Part model, mm, in its own coordinate system. A direction names the side the tool comes from. Round coordinates to 2 decimals unless told otherwise and drop trailing zeros. Loops run counter-clockwise (first coordinate to the right, second up) from the corner with the lowest first, then second, coordinate; pieces in that order, holes last.
(1) Cut at B-B on y = -24.25. List the corners of the cut face in (x, z).
(2) Mould opens along X. For faces 6 (the face through (-1.377, -16.901, 0.641)), 7 (the face through (-11, -18.5, 1)), 8 (the face through (-42.05, -4, -4)) say: +X half, -X half, draft (parallel to the pull), parting line (faces both ways), or undercut.
(3) Cut at D-D on x = -38. List the corners of the cut face in (y, z), then the cut area to 3 significant figures.
(4) Tool access for faces 1 (the face through (-33.938, -4, -4)), 2 (the face through (-40, -8.5, -4)), 3 (the face through (-49.732, -25, 1)), 4 (the face through (-43.48, -5.12, 6.23)), 5 (the face through (-31, -4, -9)): list every direction of +Z, -Z, +X, -X, +Y, -Y with a clear straight run to the whole face (end or side of a thin tool).
(5) Probe probe 1 along X at (y, z) = (-2.75, -7); probe 2 along X at (y, z) = (-3.5, 4); probe 3 along Z at (x, y) = (-55, -14). List the from-to ranges inside material, lowest first.
(6) Flat gauge pins, fed straight in: pin 1 (4 mm diameter, centred on x = -2, z = -6.5, fed in from -Y); pin 2 (1.5 mm diameter, centred on x = -37.5, z = 6, fed in from +Y); pin 3 (14 mm diameter, centred on x = -22, y = -20, fed in from -Z); pin 4 (2.5 mm diameter, centred on y = -4.5, z = -6.5, fed in from +X). Where does each tip first touch, or does it go through?
(7) Cut at A-A on z = -3.25. List the corners of the cut face in (x, y), then the cut area to 3 significant figures.
(8) Cut at C-C on z = 4.75. List the corners of the cut face in (x, y), then the cut area to 3 significant figures.
from build123d import *

# Parameters (mm, degrees)
EXTRUDE_1_DEPTH     = 1.3
SKETCH_2_R          = 6.1271e-05
SKETCH_2_R_2        = 1.854699803
CUT_EXTRUDE_1_DEPTH = 1.3
SKETCH_3_W          = 5
SKETCH_3_H          = 8.5
EXTRUDE_2_DEPTH     = 9
SKETCH_4_W          = 22.322793398
SKETCH_4_H          = 7.656611546
EXTRUDE_3_DEPTH     = 6
SKETCH_7_R          = 2.060894962
SKETCH_7_R_2        = 0.009430026
EXTRUDE_6_DEPTH     = 1.3
SKETCH_9_R          = 1.766576119
SKETCH_9_R_2        = 1.77
CUT_EXTRUDE_4_DEPTH = 13.5
SKETCH_11_R         = 2.5
EXTRUDE_7_DEPTH     = 10
SKETCH_5_R          = 3.177873229
EXTRUDE_4_DEPTH     = 10


with BuildPart() as part:
    # 草图1 → 凸台-拉伸1 (new body)
    with BuildSketch(Plane.XY):
        Polygon((-20.731582571, -20.531304637), (-20.731582571, -28.5), (-49.731582571, -28.5), (-49.731582571, -20.531304637), (-52.024986974, -18.5), (-67.347016347, -18.5), (-70.5, -15.347016347), (-70.5, 0), (0, 0), (0, -15.347016347), (-2.792647606, -18.5), (-18.700277933, -18.5), align=None)
    extrude(amount=EXTRUDE_1_DEPTH)

    # 草图2 → 切除-拉伸1 (cut)
    with BuildSketch(Plane(origin=(-0.901876225, 0, 0), x_dir=(-1, 0, 0), z_dir=(0, 0, -1))):
        with Locations((38.822404022, -18.263145779)):
            Circle(SKETCH_2_R)
        with Locations((24.094803283, -18.263145779)):
            Circle(SKETCH_2_R_2)
    extrude(amount=-CUT_EXTRUDE_1_DEPTH, mode=Mode.SUBTRACT)

    # 草图3 → 凸台-拉伸2 (add)
    with BuildSketch(Plane(origin=(0, 0, 0), x_dir=(-1, 0, 0), z_dir=(0, 0, -1))):
        with Locations((2.5, -4.25)):
            Rectangle(SKETCH_3_W, SKETCH_3_H)
        with Locations((31.437833881, -4.25)):
            Rectangle(SKETCH_3_W, SKETCH_3_H)
        with Locations((39.549598659, -4.25)):
            Rectangle(SKETCH_3_W, SKETCH_3_H)
        with Locations((67.475480729, -4.25)):
            Rectangle(SKETCH_3_W, SKETCH_3_H)
    extrude(amount=EXTRUDE_2_DEPTH)

    # 草图4 → 凸台-拉伸3 (add)
    with BuildSketch(Plane.XY.offset(1.3)):
        with Locations((-35.107201512, -24.671694227)):
            Rectangle(SKETCH_4_W, SKETCH_4_H)
    extrude(amount=EXTRUDE_3_DEPTH)

    # 草图7 → 凸台-拉伸6 (add)
    with BuildSketch(Plane(origin=(0, 0, 0), x_dir=(-1, 0, 0), z_dir=(0, 0, -1))):
        with Locations((24.996679508, -18.263145779)):
            Circle(SKETCH_7_R)
        with Locations((22.922712851, -19.688356139)):
            Circle(SKETCH_7_R_2)
    extrude(amount=-EXTRUDE_6_DEPTH)

    # 草图9 → 切除-拉伸4 (cut)
    with BuildSketch(Plane(origin=(0, 0, 0), x_dir=(-1, 0, 0), z_dir=(0, 0, -1))):
        with Locations((22.486064791, -16.932374865)):
            Circle(SKETCH_9_R)
        with Locations((47.612418274, -17.394192754)):
            Circle(SKETCH_9_R_2)
    extrude(amount=-CUT_EXTRUDE_4_DEPTH, mode=Mode.SUBTRACT)

    # 草图11 → 凸台-拉伸7 (add)
    with BuildSketch(Plane.XY.offset(1.3)):
        with Locations((-7.049667213, -4.299078236)):
            Circle(SKETCH_11_R)
        with Locations((-25.10539175, -4.501377507)):
            Circle(SKETCH_11_R)
        with Locations((-45.789989635, -4.160939668)):
            Circle(SKETCH_11_R)
        with Locations((-62.923589595, -4.217113271)):
            Circle(SKETCH_11_R)
    extrude(amount=EXTRUDE_7_DEPTH)

    # 草图5 → 凸台-拉伸4 (add)
    with BuildSketch(Plane.XY.offset(1.3)):
        with Locations((-60.836996038, -4.474043661)):
            Circle(SKETCH_5_R)
    extrude(amount=EXTRUDE_4_DEPTH)


solid = part.part
Final values:
1. outline: (-49.73, 0) - (-20.73, 0) - (-20.73, 1.3) - (-23.95, 1.3) - (-23.95, 7.3) - (-46.27, 7.3) - (-46.27, 1.3) - (-49.73, 1.3) - close
2. face 6: +X half
2. face 7: draft
2. face 8: undercut
3. outline: (-28.5, 0) - (-8.5, 0) - (-8.5, -9) - (0, -9) - (0, 1.3) - (-20.84, 1.3) - (-20.84, 7.3) - (-28.5, 7.3) - close
3. area: 159 mm2
4. face 1: -Z, +Y, -Y
4. face 2: -Z, +X, -X, -Y
4. face 3: +Z, -Z, -X, -Y
4. face 4: +Z
4. face 5: -Z, +X, -X, +Y, -Y
5. probe 1: x = -69.98 to -64.98, -42.05 to -37.05, -33.94 to -28.94, -5 to 0
5. probe 2: x = -65.32 to -57.81, -48.2 to -43.38, -27.4 to -22.81, -9.42 to -4.68
5. probe 3: z = 0 to 1.3
6. pin 1: stops at y = -8.5
6. pin 2: stops at y = -20.84
6. pin 3: stops at z = 0
6. pin 4: stops at x = 0
7. outline: (-69.98, -8.5) - (-64.98, -8.5) - (-64.98, 0) - (-69.98, 0) - close; (-42.05, -8.5) - (-37.05, -8.5) - (-37.05, 0) - (-42.05, 0) - close; (-33.94, -8.5) - (-28.94, -8.5) - (-28.94, 0) - (-33.94, 0) - close; (-5, -8.5) - (0, -8.5) - (0, 0) - (-5, 0) - close
7. area: 170 mm2
8. outline: (-63.09, -6.71) arc R3.18 ccw (long way) to (-62.48, -1.76) arc R2.5 ccw (long way) to start; circle Ø5 at (-45.79, -4.16); (-46.27, -28.5) - (-23.95, -28.5) - (-23.95, -20.84) - (-46.27, -20.84) - close; circle Ø5 at (-25.11, -4.5); circle Ø5 at (-7.05, -4.3)
8. area: 268 mm2
